Source: three-view drawing plus pictorial views. Frame: mm from the lowest corner of the part. Coordinates: 2 decimals unless noted, no trailing zeros. Write each loop counter-clockwise with the first axis right and the second up, starting at its lowest first coordinate (ties: lowest second). Pieces come first, ordered by that corner, then holes.
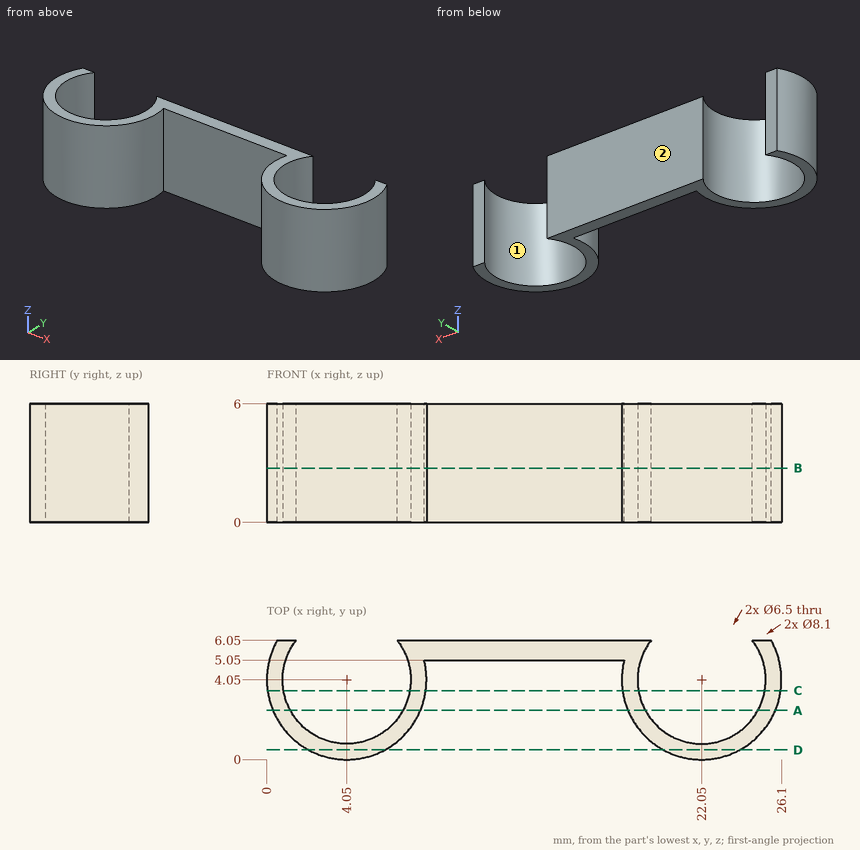
Item 1: Section query D-D, the plane y = 0.5. Return loops of the section in (x, z).
Item 2: Section query C-C, the plane y = 3.5. Return loops of the section in (x, z).
Item 3: Pin query (flat end, axial travel): pin 1 Ø1.5 at (y, z) = (1, 2.5) entering from -X; pin 2 Ø1.8 at (x, z) = (15.5, 2.5) entering from -Y; pin 3 Ø2 at (x, y) = (20, 4.5) entering from -Z. Return the tip coordinate at first contact, or that it passes through.
Item 4: Section query A-A, the plane y = 2.5. Return loops of the section in (x, z).
Item 5: Pull-direction query (X, two-part tool) for the marked faces 1 and 2; classes: released by +X, released by -X, zero draft, split by the parting line, or undercut.
Item 6: Material intervals for line 1 (X direction, y = 5, z = 4.3); line 2 (X direction, y = 2, z = 5.35); line 3 (X direction, y = 5.75, z = 3.1), sorted ascending.
Item 7: Section query B-B, the plane z = 2.75. Return loops of the section in (x, y).
The answers:
1. outline: (2.1, 0) - (6, 0) - (6, 6) - (2.1, 6) - close; (20.1, 0) - (24, 0) - (24, 6) - (20.1, 6) - close
2. outline: (0.04, 0) - (0.85, 0) - (0.85, 6) - (0.04, 6) - close; (7.25, 0) - (8.06, 0) - (8.06, 6) - (7.25, 6) - close; (18.04, 0) - (18.85, 0) - (18.85, 6) - (18.04, 6) - close; (25.25, 0) - (26.06, 0) - (26.06, 6) - (25.25, 6) - close
3. pin 1: stops at x = 0.72
3. pin 2: stops at y = 5.05
3. pin 3: passes through
4. outline: (0.31, 0) - (1.19, 0) - (1.19, 6) - (0.31, 6) - close; (6.91, 0) - (7.79, 0) - (7.79, 6) - (6.91, 6) - close; (18.31, 0) - (19.19, 0) - (19.19, 6) - (18.31, 6) - close; (24.91, 0) - (25.79, 0) - (25.79, 6) - (24.91, 6) - close
5. face 1: undercut
5. face 2: zero draft
6. line 1: x = 0.11 to 0.94, 7.16 to 7.99, 18.11 to 18.94, 25.16 to 25.99
6. line 2: x = 0.56 to 1.53, 6.57 to 7.54, 18.56 to 19.53, 24.57 to 25.54
6. line 3: x = 0.37 to 1.28, 6.82 to 19.28, 24.82 to 25.73
7. outline: (0.53, 6.05) arc R4.05 ccw (long way) to (7.97, 5.05) - (18.13, 5.05) arc R4.05 ccw (long way) to (25.57, 6.05) - (24.61, 6.05) arc R3.25 cw (long way) to (19.49, 6.05) - (6.61, 6.05) arc R3.25 cw (long way) to (1.49, 6.05) - close
